```python
from build123d import *

# Parameters (mm, degrees)
BOSS_EXTRUDE1_DEPTH = 50.8
CUT_EXTRUDE1_REACH  = 68.372
SKETCH2_R           = 3.302
SKETCH3_R           = 3.302
CUT_EXTRUDE2_DEPTH  = 67.371930249


with BuildPart() as part:
    # Sketch1 → Boss-Extrude1 (new body)
    with BuildSketch(Plane(origin=(0, 0, 0), x_dir=(1, 0, 0), z_dir=(0, 1, 0))):
        Polygon((0, 0), (0, -28.575), (31.75, -28.575), (31.75, 0), (28.575, 0), (28.575, -25.4), (3.175, -25.4), (3.175, 0), align=None)
    extrude(amount=BOSS_EXTRUDE1_DEPTH)

    # Sketch2 → Cut-Extrude1 (cut, up to next)
    with BuildSketch(Plane.XY.offset(28.575), mode=Mode.PRIVATE) as cut_extrude1_sk1:
        with Locations((15.875, 38.1)):
            Circle(SKETCH2_R)
    cut_extrude1_tool1 = extrude(cut_extrude1_sk1.sketch, amount=-CUT_EXTRUDE1_REACH, mode=Mode.PRIVATE) & part.part
    # Sketch2 → Cut-Extrude1 (cut, up to next)
    with BuildSketch(Plane.XY.offset(28.575), mode=Mode.PRIVATE) as cut_extrude1_sk2:
        with Locations((15.875, 12.7)):
            Circle(SKETCH2_R)
    cut_extrude1_tool2 = extrude(cut_extrude1_sk2.sketch, amount=-CUT_EXTRUDE1_REACH, mode=Mode.PRIVATE) & part.part
    add(cut_extrude1_tool1.solids().sort_by_distance((15.875, 38.1, 28.575))[0], mode=Mode.SUBTRACT)
    add(cut_extrude1_tool2.solids().sort_by_distance((15.875, 12.7, 28.575))[0], mode=Mode.SUBTRACT)

    # Sketch3 → Cut-Extrude2 (cut, through all)
    with BuildSketch(Plane(origin=(31.75, 0, 0), x_dir=(0, 0, -1), z_dir=(1, 0, 0))):
        with Locations((-12.7, 38.1)):
            Circle(SKETCH3_R)
        with Locations((-12.7, 12.7)):
            Circle(SKETCH3_R)
    extrude(amount=-CUT_EXTRUDE2_DEPTH, mode=Mode.SUBTRACT)


solid = part.part
```
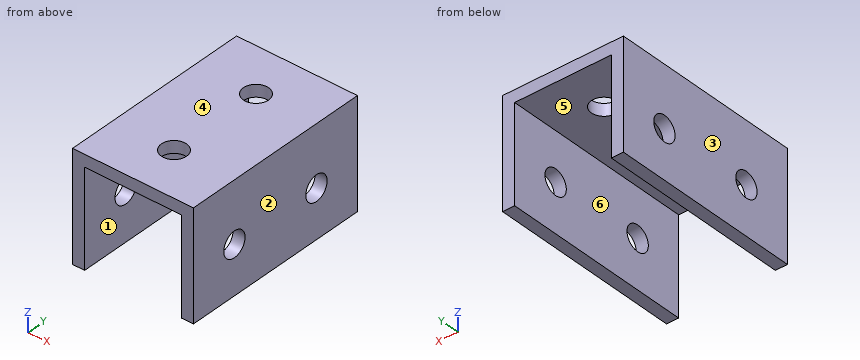
Here's how the part is built. I have some questions about the finished solid (model axes, mm). Face numbers are marked on the shaded views. A direction names the side the tool comes from. Round coordinates to 2 decimals unless told otherwise and drop trailing zeros. Order: outer loops, then holes, each group sorted by start corner. A loop starts at its lowest first (then second) coordinate and runs counter-clockwise, first axis right, second up. Notation, with made-up numbers: M 81.5,-14.5 L 112.5,-14.5 A32 cw 112.5,24.5 Z; hole C 88.25,80 d8. An arc over 180 degrees is marked long. Answer as CSV lines item,"result".
Item 1: We'd pull the mould along X, two halves only. Please class the marked faces 3, 4, 5 and 6: +X half, -X half, draft (parallel to the pull), parting line (faces both ways), or undercut.
From the geometry:
face 3,"-X half"
face 4,"draft"
face 5,"undercut"
face 6,"undercut"
Item 2: Imagine slicing it at B-B on z = 17.5. List the corners of the cut face in (x, y) for me (3 decimals).
From the geometry:
outline,"M 0,0 L 3.175,0 L 3.175,50.8 L 0,50.8 Z; M 28.575,0 L 31.75,0 L 31.75,50.8 L 28.575,50.8 Z"
Item 3: Please list where these lines run through material, in increasing order: L1, parallel to Y at x = 2.5, z = 12.7; L2, parallel to X at y = 26, z = 5 (3 decimals); L3, parallel to Z at x = 2, y = 38 (3 decimals). Write a range as [from, to].
From the geometry:
L1,"[0, 9.4], [16, 34.8], [41.4, 50.8]"
L2,"[0, 3.175], [28.575, 31.75]"
L3,"[0, 9.4], [16, 28.575]"
Item 4: For pin 1 (12.5 mm diameter, centred on x = 15, y = 13, fed in from -Z), with a flat end and sliding along its axis, tell me the tip position at first contact or that it passes through.
From the geometry:
pin 1,"z = 25.4"
Item 5: Which directions (+Z, -Z, +X, -X, +Y, -Y) give clear straight access to the entire face, cutting with the end or side of a thin tool? Please do the marked faces 1 and 2.
From the geometry:
face 1,"-Z, +Y, -Y"
face 2,"+Z, -Z, +X, +Y, -Y"
Item 6: Imagine slicing it at D-D on x = 15. List the corners of the cut face in (y, z) for me (3 decimals), and give its area (3 significant figures).
From the geometry:
outline,"M 0,25.4 L 9.516,25.4 L 9.516,28.575 L 0,28.575 Z; M 15.884,25.4 L 34.916,25.4 L 34.916,28.575 L 15.884,28.575 Z; M 41.284,25.4 L 50.8,25.4 L 50.8,28.575 L 41.284,28.575 Z"
area,"121 mm2"
Item 7: Imagine slicing it at A-A on y = 12.7. List the corners of the cut face in (x, z) for me (3 decimals), and give its area (3 significant figures).
From the geometry:
outline,"M 0,0 L 3.175,0 L 3.175,9.398 L 0,9.398 Z; M 0,16.002 L 3.175,16.002 L 3.175,25.4 L 12.573,25.4 L 12.573,28.575 L 0,28.575 Z; M 19.177,25.4 L 28.575,25.4 L 28.575,16.002 L 31.75,16.002 L 31.75,28.575 L 19.177,28.575 Z; M 28.575,0 L 31.75,0 L 31.75,9.398 L 28.575,9.398 Z"
area,"199 mm2"
Item 8: Imagine slicing it at C-C on z = 12.7. List the corners of the cut face in (x, y) for me (3 decimals), and give its area (3 significant figures).
From the geometry:
outline,"M 0,0 L 3.175,0 L 3.175,9.398 L 0,9.398 Z; M 0,16.002 L 3.175,16.002 L 3.175,34.798 L 0,34.798 Z; M 0,41.402 L 3.175,41.402 L 3.175,50.8 L 0,50.8 Z; M 28.575,0 L 31.75,0 L 31.75,9.398 L 28.575,9.398 Z; M 28.575,16.002 L 31.75,16.002 L 31.75,34.798 L 28.575,34.798 Z; M 28.575,41.402 L 31.75,41.402 L 31.75,50.8 L 28.575,50.8 Z"
area,"239 mm2"
